Build history of the part. All positions in model axes, mm. Round coordinates to 2 decimals unless told otherwise and drop trailing zeros. Write each loop counter-clockwise with the first axis right and the second up, starting at its lowest first coordinate (ties: lowest second). Pieces come first, ordered by that corner, then holes. Notation, with made-up numbers: (-22.5, 59.25) -> (6.5, 59.25) arc R9 ccw to (6.5, 73.25) -> close; hole circle Ø9 at (36, 25). An arc over 180 degrees is marked (long way). Answer in a Markdown table with one row per item.
```python
from build123d import *

# Parameters (mm, degrees)
CYLINDER044_R     = 2.6
CYLINDER044_DEPTH = 12
CYLINDER041_R     = 7
CYLINDER041_DEPTH = 6


with BuildPart() as obj1:
    # Cylinder044 → Cylinder044 (new body)
    with BuildSketch(Plane.XY.offset(13)):
        Circle(CYLINDER044_R)
    extrude(amount=CYLINDER044_DEPTH)


with BuildPart() as cut005:
    # Cylinder041 → Cylinder041 (new body)
    with BuildSketch(Plane.XY.offset(13)):
        Circle(CYLINDER041_R)
    extrude(amount=CYLINDER041_DEPTH)

    # Cut005: cut obj1
    add(obj1.part, mode=Mode.SUBTRACT)


solid = cut005.part
```
Q1. Wall check: line 1 (Y direction, x = 0, z = 16.9); line 2 (Y direction, x = -1.5, z = 15.65); line 3 (X direction, y = 0.5, z = 13.8). Give the ranges that are in metal, low to high. Write a range as [from, to].
A:
| item | result |
|---|---|
| line 1 | [-7, -2.6], [2.6, 7] |
| line 2 | [-6.84, -2.12], [2.12, 6.84] |
| line 3 | [-6.98, -2.55], [2.55, 6.98] |
Q2. Saw through at D-D on x = -3.25. Write the cut outline in (y, z).
A:
| item | result |
|---|---|
| outline | (-6.2, 13) -> (6.2, 13) -> (6.2, 19) -> (-6.2, 19) -> close |
Q3. Two-plate mould, pull along Y, no slides. Class faces 1 (the cylindrical face through (6.466, -2.681, 15.958)), 2 (the cylindrical face through (-0.338, 2.578, 15.958)), 3 (the flat face through (0, -3, 13)): released by +Y, released by -Y, zero draft, split by the parting line, or undercut.
A:
| item | result |
|---|---|
| face 1 | split by the parting line |
| face 2 | undercut |
| face 3 | zero draft |
Q4. Drop flat-ended pins along their axis: P1, Ø1, axis at y = 5.5, z = 16.5, coming from the -X side; P2, Ø1.5, axis at y = -2.5, z = 17, coming from the -X side. Give the stop position or say it passes through.
A:
| item | result |
|---|---|
| P1 | x = -4.9 |
| P2 | x = -6.78 |
Q5. Saw through at C-C on z = 16.85. Write the cut outline in (x, y).
A:
| item | result |
|---|---|
| outline | circle Ø14 at (0, 0); hole circle Ø5.2 at (0, 0) |
Q6. Saw through at A-A on x = 0. Write the cut outline in (y, z).
A:
| item | result |
|---|---|
| outline | (-7, 13) -> (-2.6, 13) -> (-2.6, 19) -> (-7, 19) -> close; (2.6, 13) -> (7, 13) -> (7, 19) -> (2.6, 19) -> close |
